CAD build for the part. Positions are in the model's coordinates, mm. A direction names the side the tool comes from. Give positions to 0.01 mm unless a question says otherwise; leave off trailing zeros. Write each loop counter-clockwise with the first axis right and the second up, starting at its lowest first coordinate (ties: lowest second). Pieces come first, ordered by that corner, then holes. Notation, with made-up numbers: (7.25, 72.25) - (63.25, 72.25) arc R17 ccw to (63.25, 83.25) - close; hole circle Ø7 at (89, -18.5). An arc over 180 degrees is marked (long way). Put each result on its own line as item: value. Start each with the question number.
1. Drop flat-ended pins along their axis: pin 1 (1.5 mm diameter, centred on x = -114, y = 209, fed in from -Z); pin 2 (5 mm diameter, centred on y = 244.5, z = -85.5, fed in from +X); pin 3 (10 mm diameter, centred on x = 193.04, y = 114.3, fed in from +Z); pin 4 (1 mm diameter, centred on x = 110.5, z = 160, fed in from +Y). Give the stop position or say it passes through.
2. Wall check: line 1 (X direction, y = 96.5, z = 173); line 2 (Z direction, x = -51, y = 80.5); line 3 (X direction, y = 113.5, z = -13.5) (1 decimal). Give the ranges that are in metal, low to high.
3. Mould opens along Y. For faces 1 (the flat face through (-3.175, 144, -203)), 2 (the cylindrical face through (-194.42, 222.4, 54.2)) say: +Y half, -Y half, draft (parallel to the pull), parting line (faces both ways), or undercut.
4. Cut at C-C on y = 38.1. Give the number of separate pieces and of enclosed holes in the cut face, and give its area (3 significant figures).
5. Tool access for faces 3 (the flat face through (166.688, 144, 112)), 4 (the cylindrical face through (188, 262.84, 54.2)), 5 (the flat face through (98, 138, -228.6)): list every direction of +Z, -Z, +X, -X, +Y, -Y with a clear straight run to the whole face (end or side of a thin tool).
6. Cut at A-A on x = 23.5. List the corners of the cut face in (y, z).
7. Cut at B-B on z = -138. List the corners of the cut face in (x, y).
from build123d import *

# Parameters (mm, degrees)
BOSS_EXTRUDE1_DEPTH = 279.4
SKETCH2_R           = 6.35
CUT_EXTRUDE1_DEPTH  = 45.72
SKETCH3_R           = 6.35
CUT_EXTRUDE2_DEPTH  = 45.72
FILLET1_R           = 2.54
CUT_EXTRUDE3_DEPTH  = 274.32
FILLET2_R           = 2.54
SKETCH6_W           = 127
SKETCH6_H           = 6.35
BOSS_EXTRUDE2_DEPTH = 25.4
SKETCH8_W           = 190.5
SKETCH8_H           = 6.35
BOSS_EXTRUDE3_DEPTH = 25.4
FILLET3_R           = 6.35


with BuildPart() as part:
    # Sketch1 → Boss-Extrude1 (new body)
    with BuildSketch(Plane(origin=(0, 0, 0), x_dir=(1, 0, 0), z_dir=(0, 1, 0))):
        Polygon((-177.8, -228.6), (-31.75, -228.6), (31.75, -228.6), (177.8, -228.6), (177.8, -69.85), (206.375, -69.85), (206.375, -38.1), (177.8, -38.1), (177.8, 228.6), (15.875, 228.6), (15.875, 257.175), (-15.875, 257.175), (-15.875, 228.6), (-177.8, 228.6), (-177.8, -38.1), (-206.375, -38.1), (-206.375, -69.85), (-177.8, -69.85), align=None)
    extrude(amount=BOSS_EXTRUDE1_DEPTH)

    # Sketch2 → Cut-Extrude1 (cut)
    with BuildSketch(Plane.XY.offset(69.85)):
        with Locations((-193.04, 38.1)):
            Circle(SKETCH2_R)
        with Locations((-193.04, 76.2)):
            Circle(SKETCH2_R)
        with Locations((-193.04, 114.3)):
            Circle(SKETCH2_R)
        with Locations((-193.04, 152.4)):
            Circle(SKETCH2_R)
        with Locations((-193.04, 190.5)):
            Circle(SKETCH2_R)
        with Locations((-193.04, 228.6)):
            Circle(SKETCH2_R)
        with Locations((-193.04, 266.7)):
            Circle(SKETCH2_R)
        with Locations((193.04, 266.7)):
            Circle(SKETCH2_R)
        with Locations((193.04, 228.6)):
            Circle(SKETCH2_R)
        with Locations((193.04, 190.5)):
            Circle(SKETCH2_R)
        with Locations((193.04, 152.4)):
            Circle(SKETCH2_R)
        with Locations((193.04, 114.3)):
            Circle(SKETCH2_R)
        with Locations((193.04, 76.2)):
            Circle(SKETCH2_R)
        with Locations((193.04, 38.1)):
            Circle(SKETCH2_R)
    extrude(amount=-CUT_EXTRUDE1_DEPTH, mode=Mode.SUBTRACT)

    # Sketch3 → Cut-Extrude2 (cut)
    with BuildSketch(Plane.ZY.offset(15.875)):
        with Locations((-243.84, 38.1)):
            Circle(SKETCH3_R)
        with Locations((-243.84, 76.2)):
            Circle(SKETCH3_R)
        with Locations((-243.84, 114.3)):
            Circle(SKETCH3_R)
        with Locations((-243.84, 152.4)):
            Circle(SKETCH3_R)
        with Locations((-243.84, 190.5)):
            Circle(SKETCH3_R)
        with Locations((-243.84, 228.6)):
            Circle(SKETCH3_R)
        with Locations((-243.84, 266.7)):
            Circle(SKETCH3_R)
    extrude(amount=-CUT_EXTRUDE2_DEPTH, mode=Mode.SUBTRACT)

    # Fillet1
    fillet1_edges = [part.edges().sort_by_distance(p)[0] for p in [
        (-206.375, 139.7, 69.85),
        (-206.375, 139.7, 38.1),
        (-15.875, 139.7, -257.175),
        (15.875, 139.7, -257.175),
        (206.375, 139.7, 38.1),
        (206.375, 139.7, 69.85),
    ]]
    fillet(fillet1_edges, radius=FILLET1_R)

    # Sketch4 → Cut-Extrude3 (cut)
    with BuildSketch(Plane(origin=(0, 279.4, 0), x_dir=(1, 0, 0), z_dir=(0, 1, 0))):
        Polygon((-3.175, 215.9), (-169.8625, 215.9), (-169.8625, 193.675), (-166.6875, 193.675), (-166.6875, 28.575), (-169.8625, 28.575), (-169.8625, 6.35), (-3.175, 6.35), (-3.175, 28.575), (-6.35, 28.575), (-6.35, 193.675), (-3.175, 193.675), align=None)
        Polygon((3.175, 28.575), (6.35, 28.575), (6.35, 193.675), (3.175, 193.675), (3.175, 215.9), (169.8625, 215.9), (169.8625, 193.675), (166.6875, 193.675), (166.6875, 28.575), (169.8625, 28.575), (169.8625, 6.35), (3.175, 6.35), align=None)
        Polygon((3.175, -193.675), (3.175, -215.9), (169.8625, -215.9), (169.8625, -193.675), (166.6875, -193.675), (166.6875, -28.575), (169.8625, -28.575), (169.8625, -6.35), (3.175, -6.35), (3.175, -28.575), (6.35, -28.575), (6.35, -193.675), align=None)
        Polygon((-3.175, -193.675), (-3.175, -215.9), (-169.8625, -215.9), (-169.8625, -193.675), (-166.6875, -193.675), (-166.6875, -28.575), (-169.8625, -28.575), (-169.8625, -6.35), (-3.175, -6.35), (-3.175, -28.575), (-6.35, -28.575), (-6.35, -193.675), align=None)
    extrude(amount=-CUT_EXTRUDE3_DEPTH, mode=Mode.SUBTRACT)

    # Fillet2
    fillet2_edges = [part.edges().sort_by_distance(p)[0] for p in [
        (-169.8625, 142.24, -215.9),
        (-3.175, 142.24, -215.9),
        (-3.175, 142.24, -6.35),
        (-169.8625, 142.24, -6.35),
        (-169.8625, 142.24, 6.35),
        (-3.175, 142.24, 6.35),
        (-3.175, 142.24, 215.9),
        (-169.8625, 142.24, 215.9),
        (3.175, 142.24, -6.35),
        (3.175, 142.24, -215.9),
        (169.8625, 142.24, -215.9),
        (169.8625, 142.24, -6.35),
        (3.175, 142.24, 6.35),
        (169.8625, 142.24, 6.35),
        (169.8625, 142.24, 215.9),
        (3.175, 142.24, 215.9),
    ]]
    fillet(fillet2_edges, radius=FILLET2_R)

    # Sketch6 → Boss-Extrude2 (add)
    with BuildSketch(Plane(origin=(177.8, 0, 0), x_dir=(0, 0, -1), z_dir=(1, 0, 0))):
        with Locations((-152.4, 276.225)):
            Rectangle(SKETCH6_W, SKETCH6_H)
    boss_extrude2 = extrude(amount=BOSS_EXTRUDE2_DEPTH)

    # Mirror1: Boss-Extrude2 across plane
    add(boss_extrude2.mirror(Plane(origin=(0, 0, 0), x_dir=(0, 0, 1), z_dir=(1, 0, 0))))

    # Sketch8 → Boss-Extrude3 (add)
    with BuildSketch(Plane(origin=(177.8, 0, 0), x_dir=(0, 0, -1), z_dir=(1, 0, 0))):
        with Locations((120.65, 276.225)):
            Rectangle(SKETCH8_W, SKETCH8_H)
    boss_extrude3 = extrude(amount=BOSS_EXTRUDE3_DEPTH)

    # Mirror2: Boss-Extrude3 across plane
    add(boss_extrude3.mirror(Plane(origin=(0, 0, 0), x_dir=(0, 0, 1), z_dir=(1, 0, 0))))

    # Fillet3
    fillet3_edges = [part.edges().sort_by_distance(p)[0] for p in [
        (177.8, 276.225, 215.9),
        (177.8, 273.05, 152.4),
        (177.8, 276.225, 88.9),
        (-177.8, 276.225, 215.9),
        (-177.8, 273.05, 152.4),
        (-177.8, 276.225, 88.9),
        (177.8, 276.225, -25.4),
        (177.8, 273.05, -120.65),
        (177.8, 276.225, -215.9),
        (-177.8, 276.225, -25.4),
        (-177.8, 273.05, -120.65),
        (-177.8, 276.225, -215.9),
    ]]
    fillet(fillet3_edges, radius=FILLET3_R)


solid = part.part
Report:
1. pin 1: stops at z = -228.6
1. pin 2: stops at x = 177.8
1. pin 3: passes through
1. pin 4: stops at y = 5.08
2. line 1: x = -177.8 to -166.69, -6.35 to 6.35, 166.69 to 177.8
2. line 2: z = -228.6 to -215.9, -6.35 to 6.35, 215.9 to 228.6
2. line 3: x = -177.8 to -169.9, -3.2 to 3.2, 169.9 to 177.8
3. face 1: draft
3. face 2: undercut
4. separate pieces: 4
4. enclosed holes: 4
4. area: 28,600 mm²
5. face 3: +Y
5. face 4: +Z, -Z
5. face 5: -Z, +X, +Y, -Y
6. outline: (0, -228.6) - (279.4, -228.6) - (279.4, -215.9) - (5.08, -215.9) - (5.08, -6.35) - (279.4, -6.35) - (279.4, 6.35) - (5.08, 6.35) - (5.08, 215.9) - (279.4, 215.9) - (279.4, 228.6) - (0, 228.6) - close
7. outline: (-203.2, 273.05) - (-184.15, 273.05) arc R6.35 cw to (-177.8, 266.7) - (-177.8, 0) - (177.8, 0) - (177.8, 266.7) arc R6.35 cw to (184.15, 273.05) - (203.2, 273.05) - (203.2, 279.4) - (166.69, 279.4) - (166.69, 5.08) - (6.35, 5.08) - (6.35, 279.4) - (-6.35, 279.4) - (-6.35, 5.08) - (-166.69, 5.08) - (-166.69, 279.4) - (-203.2, 279.4) - close
